The figure shows three views and two pictorial views of one solid part (mm, origin at its lowest corner). Answer the questions. Round coordinates to 2 decimals unless told otherwise and drop trailing zeros. Write each loop counter-clockwise with the first axis right and the second up, starting at its lowest first coordinate (ties: lowest second). Pieces come first, ordered by that corner, then holes.
Item 1: Find the intervals of material crossed by probe 1 along Y at (x, z) = (118.5, 1.9); probe 2 along Y at (x, z) = (9, 2.75); probe 3 along X at (y, z) = (24, 2.6), in increasing order.
Item 2: Find section B-B on x = 43.36. Give the vertices of the cut face in (y, z).
Item 3: Find section D-D on y = 3.75. Give the vertices of the cut face in (x, z).
Item 4: Each of these flat-tipped pins is pushed along its axis until it touches: pin 1 (2 mm diameter, centred on x = 135.75, y = 21, fed in from +Z); pin 2 (1 mm diameter, centred on y = 17.5, z = 1.5, fed in from -X); pin 3 (0.9 mm diameter, centred on x = 74.5, z = 2, fed in from +Y). Where does it stop, or does it pass through?
Item 5: Find section C-C on z = 1.3. Give the number of separate pieces and of enclosed holes in the cut face, then the cut area to 3 significant figures.
Item 6: Find section A-A on x = 118.5. Give the vertices of the cut face in (y, z).
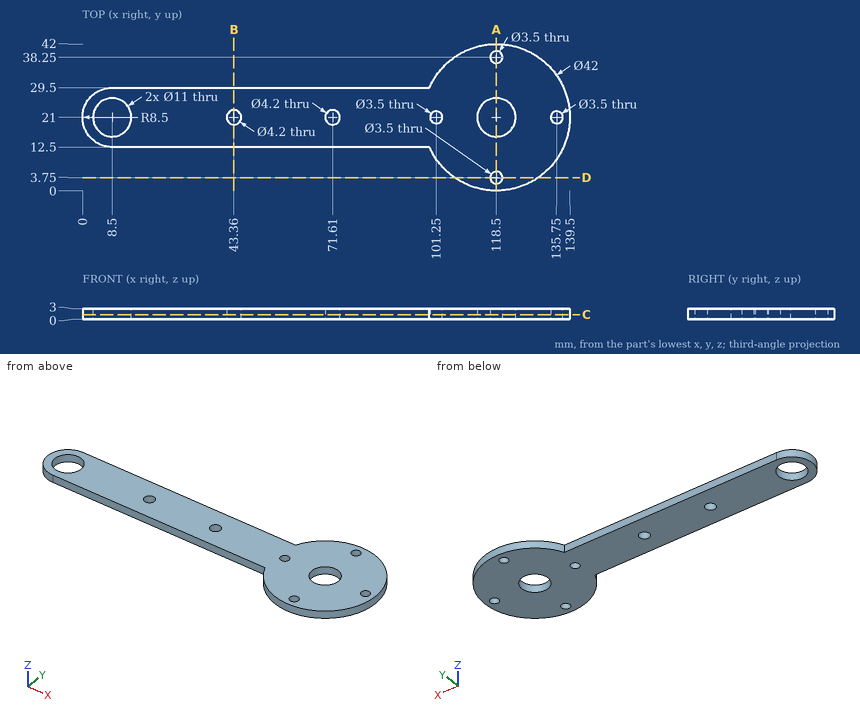
Check values:
1. probe 1: y = 0 to 2, 5.5 to 15.5, 26.5 to 36.5, 40 to 42
1. probe 2: y = 12.5 to 15.52, 26.48 to 29.5
1. probe 3: x = 0.55 to 3.89, 13.11 to 113.89, 123.11 to 139.28
2. outline: (12.5, 0) - (18.9, 0) - (18.9, 3) - (12.5, 3) - close; (23.1, 0) - (29.5, 0) - (29.5, 3) - (23.1, 3) - close
3. outline: (106.52, 0) - (116.75, 0) - (116.75, 3) - (106.52, 3) - close; (120.25, 0) - (130.48, 0) - (130.48, 3) - (120.25, 3) - close
4. pin 1: passes through
4. pin 2: stops at x = 0.55
4. pin 3: stops at y = 29.5
5. separate pieces: 1
5. enclosed holes: 8
5. area: 2,770 mm2
6. outline: (0, 0) - (2, 0) - (2, 3) - (0, 3) - close; (5.5, 0) - (15.5, 0) - (15.5, 3) - (5.5, 3) - close; (26.5, 0) - (36.5, 0) - (36.5, 3) - (26.5, 3) - close; (40, 0) - (42, 0) - (42, 3) - (40, 3) - close
